Geometry: final body of the model. Coordinates: model frame, mm. Face numbers are marked on the shaded views. A direction names the side the tool comes from. Round coordinates to 2 decimals unless told otherwise and drop trailing zeros. Loops run counter-clockwise (first coordinate to the right, second up) from the corner with the lowest first, then second, coordinate; pieces in that order, holes last. Notation, with made-up numbers: M 53,63 L 94,63 A18 cw 94,76 Z; hole C 40,73.25 d11. An arc over 180 degrees is marked long. Answer as a JSON object with one key per item and string values.
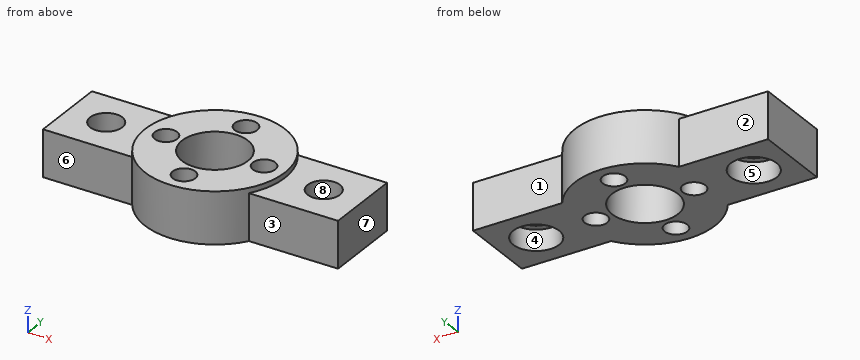
```python
from build123d import *

# Parameters (mm, degrees)
SKETCH1_R           = 10.85
SKETCH1_R_2         = 5.1
SKETCH1_R_3         = 1.75
BOSS_EXTRUDE1_DEPTH = 8
SKETCH2_R           = 3.55
BOSS_EXTRUDE3_DEPTH = 3.2
SKETCH3_R           = 2.5
BOSS_EXTRUDE4_DEPTH = 4


with BuildPart() as part:
    # Sketch1 → Boss-Extrude1 (new body)
    with BuildSketch(Plane.XY):
        Circle(SKETCH1_R)
        Circle(SKETCH1_R_2, mode=Mode.SUBTRACT)
        with Locations((-7.6, 0)):
            Circle(SKETCH1_R_3, mode=Mode.SUBTRACT)
        with Locations((0, 7.6)):
            Circle(SKETCH1_R_3, mode=Mode.SUBTRACT)
        with Locations((7.6, 0)):
            Circle(SKETCH1_R_3, mode=Mode.SUBTRACT)
        with Locations((0, -7.6)):
            Circle(SKETCH1_R_3, mode=Mode.SUBTRACT)
    extrude(amount=BOSS_EXTRUDE1_DEPTH)

    # Sketch2 → Boss-Extrude3 (add)
    with BuildSketch(Plane(origin=(0, 0, 0), x_dir=(-1, 0, 0), z_dir=(0, 0, -1))):
        with BuildLine():
            Line((-22.85, -6), (-22.85, 6))
            Line((-22.85, 6), (-9.040049779, 6))
            ThreePointArc((-9.040049779, 6), (-10.85, 0), (-9.040049779, -6))
            Line((-9.040049779, -6), (-22.85, -6))
        make_face()
        with Locations((-16.85, 0)):
            Circle(SKETCH2_R, mode=Mode.SUBTRACT)
        with BuildLine():
            Line((22.85, -6), (22.85, 6))
            Line((22.85, 6), (9.040049779, 6))
            ThreePointArc((9.040049779, 6), (10.85, 0), (9.040049779, -6))
            Line((9.040049779, -6), (22.85, -6))
        make_face()
        with Locations((16.85, 0)):
            Circle(SKETCH2_R, mode=Mode.SUBTRACT)
    extrude(amount=-BOSS_EXTRUDE3_DEPTH)

    # Sketch3 → Boss-Extrude4 (add)
    with BuildSketch(Plane.XY.offset(3.2)):
        with BuildLine():
            Line((-9.040049779, 6), (-22.85, 6))
            Line((-22.85, 6), (-22.85, -6))
            Line((-22.85, -6), (-9.040049779, -6))
            ThreePointArc((-9.040049779, -6), (-10.85, 0), (-9.040049779, 6))
        make_face()
        with Locations((-16.85, 0)):
            Circle(SKETCH3_R, mode=Mode.SUBTRACT)
        with BuildLine():
            Line((9.040049779, -6), (22.85, -6))
            Line((22.85, -6), (22.85, 6))
            Line((22.85, 6), (9.040049779, 6))
            ThreePointArc((9.040049779, 6), (10.85, 0), (9.040049779, -6))
        make_face()
        with Locations((16.85, 0)):
            Circle(SKETCH3_R, mode=Mode.SUBTRACT)
    extrude(amount=BOSS_EXTRUDE4_DEPTH)


solid = part.part
```
1) Cut plane A-A on z = 2.5. Return the cut outline in (x, y).
Geometry results:
{"outline": "M -22.85,-6 L -9.04,-6 A10.85 ccw 9.04,-6 L 22.85,-6 L 22.85,6 L 9.04,6 A10.85 ccw -9.04,6 L -22.85,6 Z; hole C -16.85,0 d7.1; hole C -7.6,0 d3.5; hole C 0,0 d10.2; hole C 0,-7.6 d3.5; hole C 0,7.6 d3.5; hole C 7.6,0 d3.5; hole C 16.85,0 d7.1"}
2) Cut plane D-D on y = -4. Return the cut outline in (x, z).
Geometry results:
{"outline": "M -22.85,0 L -3.16,0 L -3.16,8 L -10.09,8 L -10.09,7.2 L -22.85,7.2 Z; M 3.16,0 L 22.85,0 L 22.85,7.2 L 10.09,7.2 L 10.09,8 L 3.16,8 Z"}
3) Cut plane C-C on x = 16.85. Return the cut outline in (y, z).
Geometry results:
{"outline": "M -6,0 L -3.55,0 L -3.55,3.2 L -2.5,3.2 L -2.5,7.2 L -6,7.2 Z; M 2.5,3.2 L 3.55,3.2 L 3.55,0 L 6,0 L 6,7.2 L 2.5,7.2 Z"}
4) Set-up query: the marked faces 1, 2, 3 and 4. Return all of +Z, -Z, +X, -X, +Y, -Y with unobstructed straight access to the full face (end or side cutting, diameter ignored); none if empty.
Geometry results:
{"face 1": "+Z, -Z, +X, +Y", "face 2": "+Z, -Z, -X, +Y", "face 3": "+Z, -Z, +X, -Y", "face 4": "-Z"}
5) Cut plane B-B on x = 0. Return the cut outline in (y, z), and give its area (3 significant figures).
Geometry results:
{"outline": "M -10.85,0 L -9.35,0 L -9.35,8 L -10.85,8 Z; M -5.85,0 L -5.1,0 L -5.1,8 L -5.85,8 Z; M 5.1,0 L 5.85,0 L 5.85,8 L 5.1,8 Z; M 9.35,0 L 10.85,0 L 10.85,8 L 9.35,8 Z", "area": "36.0 mm2"}
6) Line query: probe 1 along Y at (x, z) = (0, 5.75); probe 2 along Y at (x, z) = (-1.5, 1.5); probe 3 along Y at (x, z) = (-16.85, 1.45). Output: solid intervals per line, ascending.
Geometry results:
{"probe 1": "-10.85 to -9.35, -5.85 to -5.1, 5.1 to 5.85, 9.35 to 10.85", "probe 2": "-10.75 to -8.5, -6.7 to -4.87, 4.87 to 6.7, 8.5 to 10.75", "probe 3": "-6 to -3.55, 3.55 to 6"}
7) First-contact query: pin 1 (8 mm diameter, centred on x = 16.85, y = 0, fed in from +Z); pin 2 (1 mm diameter, centred on y = 8, z = 3.5, fed in from -X); pin 3 (6.5 mm diameter, centred on x = -16.85, y = 0, fed in from -Z); pin 4 (3 mm diameter, centred on x = 7.6, y = 0, fed in from +Z). Flat tips, straight axial feed; report the tip coordinate or a pass-through.
Geometry results:
{"pin 1": "z = 7.2", "pin 2": "x = -7.84", "pin 3": "z = 3.2", "pin 4": "through"}
8) Pull-direction query (Y, two-part tool) for the marked faces 5, 6, 7 and 8; classes: +Y half, -Y half, draft (parallel to the pull), parting line (faces both ways), or undercut.
Geometry results:
{"face 5": "undercut", "face 6": "-Y half", "face 7": "draft", "face 8": "undercut"}
